Source: three-view drawing plus pictorial views. Frame: mm from the lowest corner of the part. Give positions to 0.01 mm unless a question says otherwise; leave off trailing zeros. Write each loop counter-clockwise with the first axis right and the second up, starting at its lowest first coordinate (ties: lowest second). Pieces come first, ordered by that corner, then holes.
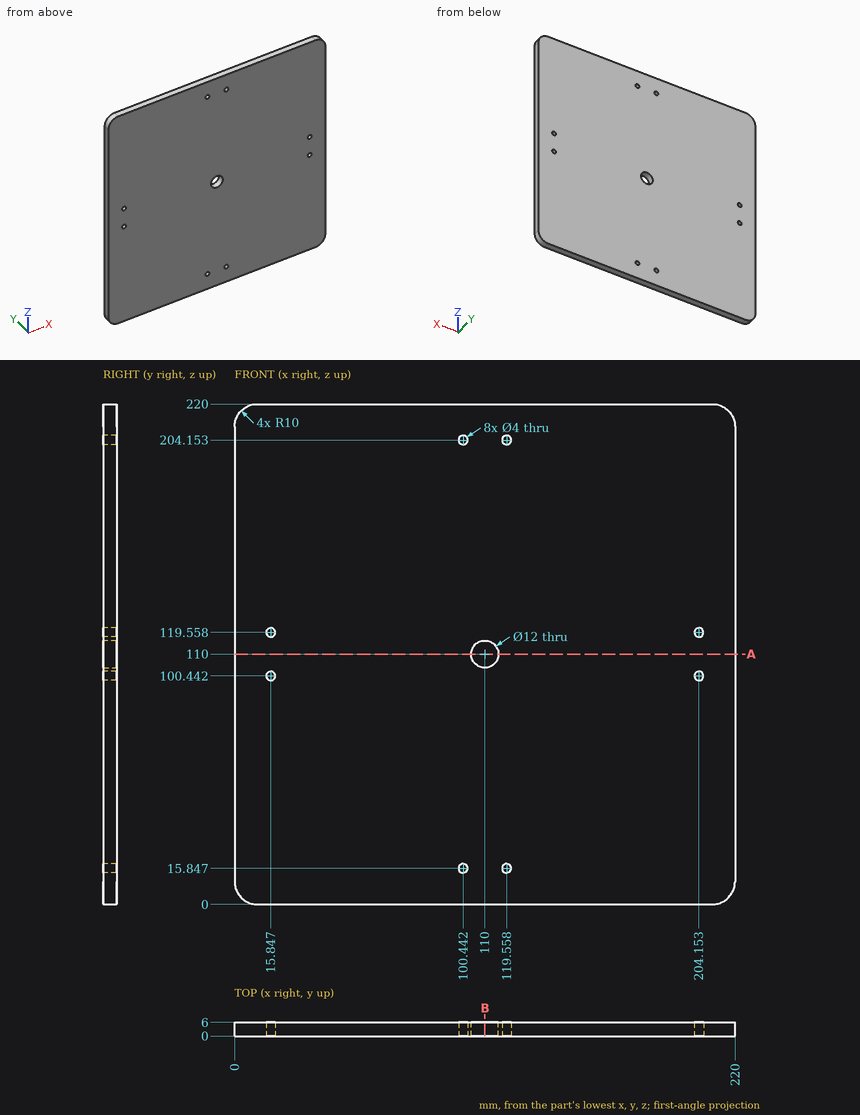
Q1. Ray query, line 1 along Z through (x, y) = (107, 5.1). Return the intervals inside material, ascending.
Filled sheet:
line 1: z = 0 to 104.8, 115.2 to 220
Q2. Section B-B on x = 110. Output: boundary loops of the cut face in (y, z), plus the area to 3 significant figures.
Filled sheet:
outline: (0, 0) - (6, 0) - (6, 104) - (0, 104) - close; (0, 116) - (6, 116) - (6, 220) - (0, 220) - close
area: 1,250 mm2
Q3. Pin query (flat end, axial travel): P1, Ø2.5, axis at x = 15.85, z = 100.44, coming from the +Y side. Return the tip coordinate at first contact, or that it passes through.
Filled sheet:
P1: passes through
Q4. Section A-A on z = 110. Output: boundary loops of the cut face in (x, y).
Filled sheet:
outline: (0, 0) - (104, 0) - (104, 6) - (0, 6) - close; (116, 0) - (220, 0) - (220, 6) - (116, 6) - close
